The listing builds one solid part. Answer for the finished solid, in the listing's coordinates (mm). A direction names the side the tool comes from. Give positions to 0.01 mm unless a question says otherwise; leave off trailing zeros. Loops run counter-clockwise (first coordinate to the right, second up) from the corner with the lowest first, then second, coordinate; pieces in that order, holes last. Notation, with made-up numbers: (59.25, 14.25) - (64.25, 14.25) arc R36 ccw to (64.25, 52.25) - close; hole circle Ø3 at (22.5, -4.75). An arc over 180 degrees is marked (long way). Write item = value, one per line. Start each with the question number.
1) The part is cut by section B-B on y = 11.5. Write down the section's boundary in (x, z), plus the area to 3 significant figures.
2) Which of the six approach directions +Z, -Z, +X, -X, +Y, -Y give full straight-line access (tool end or side, diameter ignored) to faces 4 (the flat face through (117, 53, 1)), 5 (the flat face through (59, 14, 2)), 6 (the flat face through (60, 1, 1)), 7 (the flat face through (118, 20, 1))?
3) The mould has two halves that part along X. Classify faces 1 (the flat face through (120, 5, 1)), 2 (the flat face through (115, 0, 1)), 3 (the flat face through (55, 57, 1)): +X half, -X half, draft (parallel to the pull), parting line (faces both ways), or undercut.
4) Consider probe 1 along Y at (x, z) = (90.5, 2.5); probe 2 along X at (y, z) = (24.5, 1.4); probe 3 along Y at (x, z) = (82, 1.6). Determine where each line is inside the solid, lowest interval first.
5) Flat-ended cylindrical pins translate along their axes: P1, Ø0.9, axis at y = 59, z = 2, coming from the +X side; P2, Ø1.5, axis at x = 118.5, z = 2, coming from the +Y side; P3, Ø0.9, axis at x = 5, z = 2, coming from the -Y side. Find the tip coordinate at first contact, or state that the pin passes through.
6) The part is cut by section C-C on x = 13.5. Write down the section's boundary in (y, z).
7) The part is cut by section A-A on x = 74. Write down the section's boundary in (y, z), plus the area to 3 significant figures.
from build123d import *

# Parameters (mm, degrees)
BOSS_EXTRUDE1_DEPTH = 3
SKETCH2_W           = 80
SKETCH2_H           = 15
CUT_EXTRUDE1_DEPTH  = 10


with BuildPart() as part:
    # Sketch1 → Boss-Extrude1 (new body)
    with BuildSketch(Plane.XY):
        Polygon((120, 0), (120, 10), (117, 10), (117, 20), (120, 20), (120, 30), (117, 30), (117, 40), (120, 40), (120, 50), (117, 50), (117, 57), (110, 57), (110, 60), (100, 60), (100, 57), (90, 57), (90, 60), (80, 60), (80, 57), (70, 57), (70, 60), (60, 60), (60, 57), (50, 57), (50, 60), (40, 60), (40, 57), (30, 57), (30, 60), (20, 60), (20, 57), (10, 57), (10, 60), (0, 60), (0, 50), (3, 50), (3, 40), (0, 40), (0, 30), (3, 30), (3, 20), (0, 20), (0, 10), (3, 10), (3, 3), (10, 3), (10, 0), (20, 0), (20, 3), (30, 3), (30, 0), (40, 0), (40, 3), (50, 3), (50, 0), (60, 0), (60, 3), (70, 3), (70, 0), (80, 0), (80, 3), (90, 3), (90, 0), (100, 0), (100, 3), (110, 3), (110, 0), align=None)
    extrude(amount=BOSS_EXTRUDE1_DEPTH)

    # Sketch2 → Cut-Extrude1 (cut)
    with BuildSketch(Plane.XY.offset(3)):
        with Locations((60, 21.5)):
            Rectangle(SKETCH2_W, SKETCH2_H)
    extrude(amount=-CUT_EXTRUDE1_DEPTH, mode=Mode.SUBTRACT)


solid = part.part
Answer below:
q1.outline = (0, 0) - (117, 0) - (117, 3) - (0, 3) - close
q1.area = 351 mm2
q2.face_4 = +Z, -Z, +X, +Y
q2.face_5 = +Z, -Z
q2.face_6 = +Z, -Z, -Y
q2.face_7 = +Z, -Z, +X
q3.face_1 = +X half
q3.face_2 = draft
q3.face_3 = undercut
q4.probe_1 = 0 to 14, 29 to 57
q4.probe_2 = 3 to 20, 100 to 120
q4.probe_3 = 3 to 14, 29 to 60
q5.P1 = 110
q5.P2 = 50
q5.P3 = 3
q6.outline = (0, 0) - (57, 0) - (57, 3) - (0, 3) - close
q7.outline = (0, 0) - (14, 0) - (14, 3) - (0, 3) - close; (29, 0) - (57, 0) - (57, 3) - (29, 3) - close
q7.area = 126 mm2
